```python
from build123d import *

# Parameters (mm, degrees)
SKETCH1_R           = 0.75
SKETCH1_R_2         = 0.5
BOSS_EXTRUDE1_DEPTH = 2


with BuildPart() as part:
    # Sketch1 → Boss-Extrude1 (new body)
    with BuildSketch(Plane.XY):
        with BuildLine():
            Line((12.2, 4), (16.2, 4))
            Line((16.2, 4), (16.2, 2))
            ThreePointArc((16.2, 2), (15.614213562, 0.585786438), (14.2, 0))
            Line((14.2, 0), (2, 0))
            ThreePointArc((2, 0), (0.585786438, 0.585786438), (0, 2))
            Line((0, 2), (0, 4))
            Line((0, 4), (4, 4))
            Line((4, 4), (4, 6))
            Line((4, 6), (0, 6))
            Line((0, 6), (0, 9.205))
            ThreePointArc((0, 9.205), (1.464466094, 12.740533906), (5, 14.205))
            Line((5, 14.205), (11.2, 14.205))
            ThreePointArc((11.2, 14.205), (14.735533906, 12.740533906), (16.2, 9.205))
            Line((16.2, 9.205), (16.2, 6))
            Line((16.2, 6), (12.2, 6))
            Line((12.2, 6), (12.2, 4))
        make_face()
        with Locations((13.45, 2)):
            Circle(SKETCH1_R, mode=Mode.SUBTRACT)
        with Locations((13.2, 11.205)):
            Circle(SKETCH1_R_2, mode=Mode.SUBTRACT)
        with Locations((10.2, 7.25)):
            Circle(SKETCH1_R, mode=Mode.SUBTRACT)
        with Locations((6, 7.25)):
            Circle(SKETCH1_R, mode=Mode.SUBTRACT)
        with Locations((3, 11.205)):
            Circle(SKETCH1_R_2, mode=Mode.SUBTRACT)
        with Locations((2.75, 2)):
            Circle(SKETCH1_R, mode=Mode.SUBTRACT)
    extrude(amount=BOSS_EXTRUDE1_DEPTH)


solid = part.part
```
Check sheet for the modelled part. Datum: model origin and axes. Units: mm. A direction names the side the tool comes from. Give positions to 0.01 mm unless a question says otherwise; leave off trailing zeros. Loops run counter-clockwise (first coordinate to the right, second up) from the corner with the lowest first, then second, coordinate; pieces in that order, holes last. Notation, with made-up numbers: M 29,-6.5 L 74,-6.5 A27 cw 74,24.5 Z; hole C -3,-33 d6. An arc over 180 degrees is marked long. Answer in a Markdown table with one row per item.
1) Mould release check, pull along Y, two halves, no side actions. Record for faces 1 (the face through (1.426, 12.701, 0.986)), 2 (the face through (2, 6, 1)), 3 (the face through (8, 7, 0)): released by +Y, released by -Y, zero draft, split by the parting line, or undercut.
Solutions:
| item | result |
|---|---|
| face 1 | released by +Y |
| face 2 | undercut |
| face 3 | zero draft |
2) Cross-section at D-D (x = 1.75). Enter the section's corners in (y, z), plus the area to 3 significant figures.
Solutions:
| item | result |
|---|---|
| outline | M 0.02,0 L 4,0 L 4,2 L 0.02,2 Z; M 6,0 L 13,0 L 13,2 L 6,2 Z |
| area | 22.0 mm^2 |
3) Cross-section at A-A (y = 7.25). Enter the section's corners in (x, z), plus the area to 3 significant figures.
Solutions:
| item | result |
|---|---|
| outline | M 0,0 L 5.25,0 L 5.25,2 L 0,2 Z; M 6.75,0 L 9.45,0 L 9.45,2 L 6.75,2 Z; M 10.95,0 L 16.2,0 L 16.2,2 L 10.95,2 Z |
| area | 26.4 mm^2 |
4) Thickness scan on line 1 (Y direction, x = 6, z = 1.45) (3 decimals); line 2 (Y direction, x = 2.75, z = 0.8); line 3 (X direction, y = 11, z = 0.6). Record the ranges inside material, lowest first.
Solutions:
| item | result |
|---|---|
| line 1 | y = 0 to 6.5, 8 to 14.205 |
| line 2 | y = 0 to 1.25, 2.75 to 4, 6 to 10.77, 11.64 to 13.67 |
| line 3 | x = 0.33 to 2.54, 3.46 to 12.74, 13.66 to 15.87 |
5) Tool access check on faces 4 (the face through (5.25, 7.28, 0.99)), 5 (the face through (4, 5, 1)), 6 (the face through (14, 4, 1)). Record the directions out of +Z, -Z, +X, -X, +Y, -Y that give a thin tool (end or side, any length) a straight path to the whole face; none if there is none.
Solutions:
| item | result |
|---|---|
| face 4 | +Z, -Z |
| face 5 | +Z, -Z, -X |
| face 6 | +Z, -Z, +X |
6) Depth check by flat-ended pin: pin 1 (1 mm diameter, centred on x = 4, z = 0.5, fed in from +Y). Enter the tip coordinate at first touch or a pass-through.
Solutions:
| item | result |
|---|---|
| pin 1 | stops at y = 14.18 |
7) Cross-section at C-C (z = 0.2). Enter the section's corners in (x, y) (3 decimals), plus the area to 3 significant figures.
Solutions:
| item | result |
|---|---|
| outline | M 0,2 A2 ccw 2,0 L 14.2,0 A2 ccw 16.2,2 L 16.2,4 L 12.2,4 L 12.2,6 L 16.2,6 L 16.2,9.205 A5 ccw 11.2,14.205 L 5,14.205 A5 ccw 0,9.205 L 0,6 L 4,6 L 4,4 L 0,4 Z; hole C 2.75,2 d1.5; hole C 3,11.205 d1; hole C 6,7.25 d1.5; hole C 10.2,7.25 d1.5; hole C 13.45,2 d1.5; hole C 13.2,11.205 d1 |
| area | 193 mm^2 |
8) Cross-section at B-B (x = 13.2). Enter the section's corners in (y, z) (3 decimals), plus the area to 3 significant figures.
Solutions:
| item | result |
|---|---|
| outline | M 0,0 L 1.293,0 L 1.293,2 L 0,2 Z; M 2.707,0 L 4,0 L 4,2 L 2.707,2 Z; M 6,0 L 10.705,0 L 10.705,2 L 6,2 Z; M 11.705,0 L 13.788,0 L 13.788,2 L 11.705,2 Z |
| area | 18.7 mm^2 |
